Part model, mm, in its own coordinate system. Round coordinates to 2 decimals unless told otherwise and drop trailing zeros. Write each loop counter-clockwise with the first axis right and the second up, starting at its lowest first coordinate (ties: lowest second). Pieces come first, ordered by that corner, then holes. Notation, with made-up numbers: M -38.5,-18 L -17.5,-18 A10 ccw -17.5,-14 Z; hole C 83,9 d4. An arc over 180 degrees is marked long. One line per question, with ' | ' between items. Start each with the question number.
1) Drop flat-ended pins along their axis: pin 1 Ø3 at (x, z) = (-18, -36) entering from -Y; pin 2 Ø3.5 at (x, z) = (-24.91, -37.29) entering from +Y. Give the stop position or say it passes through.
2) Saw through at A-A (z = 0.5). List the corners of the cut face in (x, y).
3) Wall check: probe 1 along Z at (x, y) = (-25, 0.5); probe 2 along X at (y, z) = (3.25, -1); probe 3 along Z at (x, y) = (-44, 8.75). Give the ranges that are in metal, low to high. Write a range as [from, to].
4) Mould opens along Z. For faces 1 (the face through (-22.29, 5.92, -20.12)), 2 (the face through (3.089, 6, -19)), 3 (the face through (-25, 6, -47.293)), 4 (the face through (-7.51, 5.92, -34.61)) say: pulls with the +Z half, pulls with the -Z half, needs draft (parallel to the pull), parting line crosses it, or undercut.
5) Saw through at C-C (x = -6). List the corners of the cut face in (y, z).
6) Saw through at B-B (y = 4.5). Give the number of separate pieces and of enclosed holes in the cut face, plus the area to 3 significant figures.
```python
from build123d import *

# Parameters (mm, degrees)
SKETCH1_W           = 56
SKETCH1_H           = 56
SKETCH1_R           = 2.75
BOSS_EXTRUDE2_DEPTH = 12


with BuildPart() as part:
    # Sketch1 → Boss-Extrude2 (new body)
    with BuildSketch(Plane(origin=(0, 0, 0), x_dir=(1, 0, 0), z_dir=(0, 1, 0))):
        with Locations((-24.911392405, 19.293363463)):
            Rectangle(SKETCH1_W, SKETCH1_H)
        with Locations((-42.911392405, 37.293363463)):
            Circle(SKETCH1_R, mode=Mode.SUBTRACT)
        with Locations((-24.911392405, 37.293363463)):
            Circle(SKETCH1_R, mode=Mode.SUBTRACT)
        with Locations((-6.911392405, 37.293363463)):
            Circle(SKETCH1_R, mode=Mode.SUBTRACT)
        with Locations((-24.911392405, 19.293363463)):
            Circle(SKETCH1_R, mode=Mode.SUBTRACT)
        with Locations((-6.911392405, 19.293363463)):
            Circle(SKETCH1_R, mode=Mode.SUBTRACT)
        with Locations((-24.911392405, 1.293363463)):
            Circle(SKETCH1_R, mode=Mode.SUBTRACT)
        with Locations((-6.911392405, 1.293363463)):
            Circle(SKETCH1_R, mode=Mode.SUBTRACT)
        with Locations((-42.911392405, 19.293363463)):
            Circle(SKETCH1_R, mode=Mode.SUBTRACT)
        with Locations((-42.911392405, 1.293363463)):
            Circle(SKETCH1_R, mode=Mode.SUBTRACT)
    extrude(amount=BOSS_EXTRUDE2_DEPTH)


solid = part.part
```
Answer key:
1) pin 1: stops at y = 0 | pin 2: passes through
2) outline: M -52.91,0 L -45,0 L -45,12 L -52.91,12 Z; M -40.83,0 L -27,0 L -27,12 L -40.83,12 Z; M -22.83,0 L -9,0 L -9,12 L -22.83,12 Z; M -4.83,0 L 3.09,0 L 3.09,12 L -4.83,12 Z
3) probe 1: z = [-47.29, -40.04], [-34.54, -22.04], [-16.54, -4.04], [1.46, 8.71] | probe 2: x = [-52.91, -45.65], [-40.18, -27.65], [-22.18, -9.65], [-4.18, 3.09] | probe 3: z = [-47.29, -39.82], [-34.77, -21.82], [-16.77, -3.82], [1.23, 8.71]
4) face 1: undercut | face 2: needs draft | face 3: pulls with the -Z half | face 4: undercut
5) outline: M 0,-47.29 L 12,-47.29 L 12,-39.89 L 0,-39.89 Z; M 0,-34.7 L 12,-34.7 L 12,-21.89 L 0,-21.89 Z; M 0,-16.7 L 12,-16.7 L 12,-3.89 L 0,-3.89 Z; M 0,1.3 L 12,1.3 L 12,8.71 L 0,8.71 Z
6) separate pieces: 1 | enclosed holes: 9 | area: 2,920 mm2
